from build123d import *

# Parameters (mm, degrees)
SKICA1_W                = 85.1
SKICA1_H                = 61.1
SKICA1_W_2              = 81.5
SKICA1_H_2              = 57.5
P_IDAT_VYSUNUT_M1_DEPTH = 35
SKICA2_W                = 101.1
SKICA2_H                = 61.1
P_IDAT_VYSUNUT_M2_DEPTH = 1.8


with BuildPart() as part:
    # Skica1 → Přidat vysunutím1 (new body)
    with BuildSketch(Plane(origin=(0, 0, 0), x_dir=(1, 0, 0), z_dir=(0, 1, 0))):
        with Locations((40.75, 28.75)):
            Rectangle(SKICA1_W, SKICA1_H)
        with Locations((40.75, 28.75)):
            Rectangle(SKICA1_W_2, SKICA1_H_2, mode=Mode.SUBTRACT)
    extrude(amount=P_IDAT_VYSUNUT_M1_DEPTH)

    # Skica2 → Přidat vysunutím2 (add)
    with BuildSketch(Plane.XZ):
        with Locations((40.75, -28.75)):
            Rectangle(SKICA2_W, SKICA2_H)
    extrude(amount=P_IDAT_VYSUNUT_M2_DEPTH)


solid = part.part
Design review of the part built by this model. Coordinates are the model's own, in mm. A direction names the side the tool comes from. Round coordinates to 2 decimals unless told otherwise and drop trailing zeros. Write each loop counter-clockwise with the first axis right and the second up, starting at its lowest first coordinate (ties: lowest second). Pieces come first, ordered by that corner, then holes. Notation, with made-up numbers: (30, -6.75) -> (81, -6.75) arc R22 cw to (81, 21.25) -> close; hole circle Ø4 at (-15.75, 11). An arc over 180 degrees is marked (long way). One line per question, with ' | ' between items.
(1) Draft analysis for pull direction Z (two halves, no side actions). For faces 1 (the flat face through (40, 17, -59.3)), 2 (the flat face through (40, 17, -57.5)), 3 (the flat face through (81.5, 17, -28)), 4 (the flat face through (40, 17, 1.8)), state which applies: released by +Z, released by -Z, zero draft, split by the parting line, or undercut.
Result sheet:
face 1: released by -Z | face 2: undercut | face 3: undercut | face 4: released by +Z
(2) Wall thickness on line 1 (X direction, y = 17, z = -14.5); line 2 (Z direction, x = 20, y = 21); line 3 (Y direction, x = 69, z = -37): over which ranges is each line inside the solid? List them lowest first. Write a range as [from, to].
Result sheet:
line 1: [-1.8, 0], [81.5, 83.3] | line 2: [-59.3, -57.5], [0, 1.8] | line 3: [-1.8, 0]
(3) Machinability: for faces 5 (the flat face through (40, 17, 0)), 6 (the flat face through (83.3, 17, -28)), 7 (the flat face through (-6, 0, -28)), which of the approach directions +Z, -Z, +X, -X, +Y, -Y give a long, thin tool a straight path to every point of the face, cutting with its end or side? Answer none if there is none.
Result sheet:
face 5: +Y | face 6: +Z, -Z, +X, +Y | face 7: +Z, -Z, -X, +Y
(4) Insertion check: P1, Ø4, axis at x = 47.5, z = -7, coming from the +Y side; P2, Ø17.5, axis at y = 13.5, z = -29.5, coming from the +X side; P3, Ø8, axis at y = 12.5, z = -53, coming from the -X side. Each pin has a flat end and moves straight along its axis. Give the tip position at first contact, or say it passes through.
Result sheet:
P1: y = 0 | P2: x = 83.3 | P3: x = -1.8
(5) Take a section at B-B, the plane z = -8.5. State the section outline as (x, y) points, and give its area (3 significant figures).
Result sheet:
outline: (-9.8, -1.8) -> (91.3, -1.8) -> (91.3, 0) -> (83.3, 0) -> (83.3, 35) -> (81.5, 35) -> (81.5, 0) -> (0, 0) -> (0, 35) -> (-1.8, 35) -> (-1.8, 0) -> (-9.8, 0) -> close | area: 308 mm2
(6) Take a section at C-C, the plane x = 65. State the section outline as (y, z) points, and give its area (3 significant figures).
Result sheet:
outline: (-1.8, -59.3) -> (35, -59.3) -> (35, -57.5) -> (0, -57.5) -> (0, 0) -> (35, 0) -> (35, 1.8) -> (-1.8, 1.8) -> close | area: 236 mm2
(7) Take a section at A-A, the plane y = 19. State the section outline as (x, z) points, and give its area (3 significant figures).
Result sheet:
outline: (-1.8, -59.3) -> (83.3, -59.3) -> (83.3, 1.8) -> (-1.8, 1.8) -> close; hole (0, -57.5) -> (81.5, -57.5) -> (81.5, 0) -> (0, 0) -> close | area: 513 mm2
